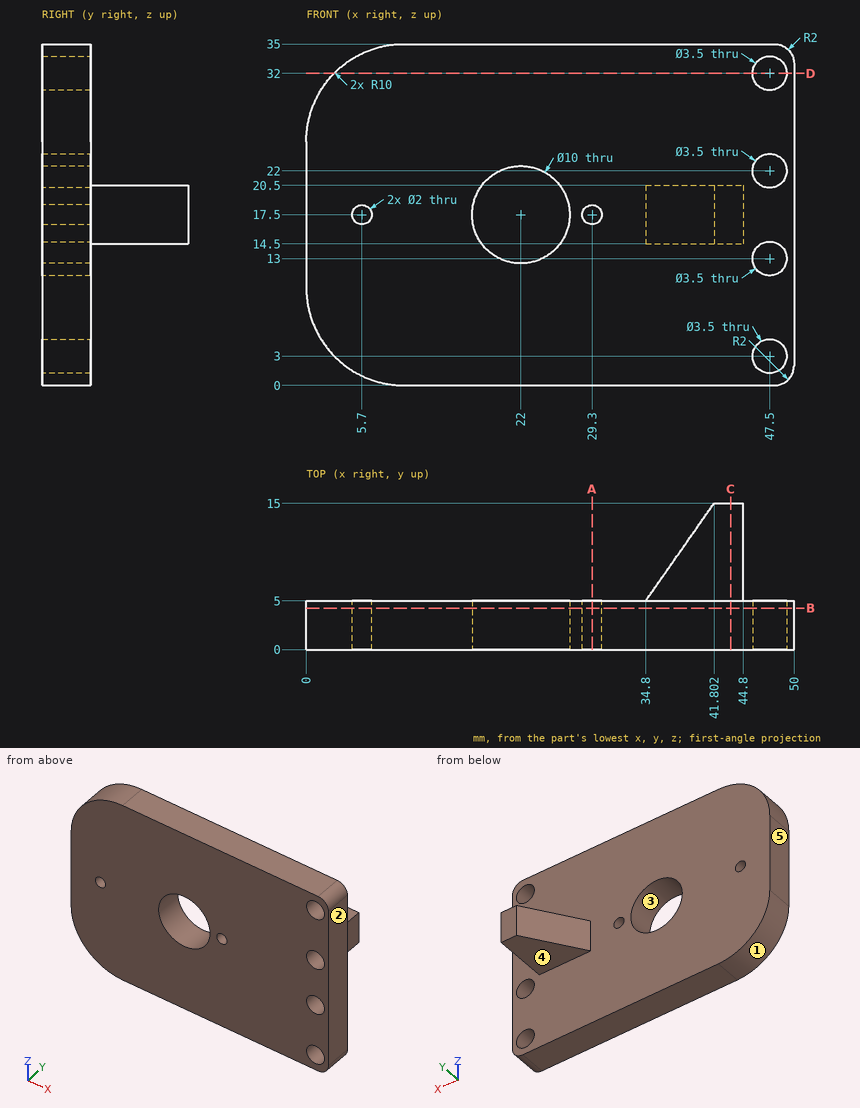
Check sheet for the drawn part. Datum: minimum x, y, z corner. Units: mm. A direction names the side the tool comes from. Coordinates: 2 decimals unless noted, no trailing zeros. Write each loop counter-clockwise with the first axis right and the second up, starting at its lowest first coordinate (ties: lowest second). Pieces come first, ordered by that corner, then holes. Notation, with made-up numbers: (33, 23) - (50, 23) arc R12 ccw to (50, 46) - close; hole circle Ø2 at (-34.75, -36). An arc over 180 degrees is marked (long way). Answer as a JSON object with one key per item and string values.
(1) Mould release check, pull along Z, two halves, no side actions. Record for the marked faces 1, 2 and 3: pulls with the +Z half, pulls with the -Z half, needs draft (parallel to the pull), parting line crosses it, or undercut.
Report:
{"face 1": "pulls with the -Z half", "face 2": "needs draft", "face 3": "undercut"}
(2) Tool access check on the marked faces 4 and 5. Record the directions out of +Z, -Z, +X, -X, +Y, -Y that give a thin tool (end or side, any length) a straight path to the whole face; none if there is none.
Report:
{"face 4": "-Z, +X, -X, +Y", "face 5": "+Z, -Z, -X, +Y, -Y"}
(3) Cross-section at D-D on z = 32. Record the cut outline in (x, y), plus the area to 3 significant figures.
Report:
{"outline": "(2.86, 0) - (45.75, 0) - (45.75, 5) - (2.86, 5) - close; (49.25, 0) - (50, 0) - (50, 5) - (49.25, 5) - close", "area": "218 mm^2"}
(4) Gauge pin test, flat ends, axial feed: pin 1 Ø1.8 at (y, z) = (11.5, 16) entering from +X; pin 2 Ø10 at (x, z) = (17, 6) entering from +Y; pin 3 Ø8 at (x, y) = (38, 10) entering from +Z; pin 4 Ø8 at (y, z) = (8, 7.5) entering from +X. Record the tip position at first contact, or that the pin passes through.
Report:
{"pin 1": "x = 44.8", "pin 2": "y = 5", "pin 3": "z = 20.5", "pin 4": "x = 50"}
(5) Thickness scan on line 1 along X through (y, z) = (2.9, 17.5); line 2 along X through (y, z) = (3.4, 13); line 3 along Y through (x, z) = (46.5, 9). Record the ranges inside material, lowest first.
Report:
{"line 1": "0 to 4.7, 6.7 to 17, 27 to 28.3, 30.3 to 50", "line 2": "0 to 19.82, 24.18 to 45.75, 49.25 to 50", "line 3": "0 to 5"}
(6) Cross-section at B-B on y = 4.25. Record the cut outline in (x, z), plus the area to 3 significant figures.
Report:
{"outline": "(0, 10) arc R10 ccw to (10, 0) - (48, 0) arc R2 ccw to (50, 2) - (50, 33) arc R2 ccw to (48, 35) - (10, 35) arc R10 ccw to (0, 25) - close; hole circle Ø2 at (5.7, 17.5); hole circle Ø10 at (22, 17.5); hole circle Ø2 at (29.3, 17.5); hole circle Ø3.5 at (47.5, 3); hole circle Ø3.5 at (47.5, 13); hole circle Ø3.5 at (47.5, 22); hole circle Ø3.5 at (47.5, 32)", "area": "1,580 mm^2"}
(7) Cross-section at A-A on x = 29.3. Record the cut outline in (y, z).
Report:
{"outline": "(0, 0) - (5, 0) - (5, 16.5) - (0, 16.5) - close; (0, 18.5) - (5, 18.5) - (5, 35) - (0, 35) - close"}
(8) Cross-section at C-C on x = 43.5. Record the cut outline in (y, z).
Report:
{"outline": "(0, 0) - (5, 0) - (5, 14.5) - (15, 14.5) - (15, 20.5) - (5, 20.5) - (5, 35) - (0, 35) - close"}
